```python
from build123d import *

# Parameters (mm, degrees)
RESSALTO_EXTRUS_O1_DEPTH      = 13.75
RESSALTO_EXTRUS_O1_DEPTH_BACK = 13.75
CORTE_EXTRUS_O1_DEPTH         = 13.75
CORTE_EXTRUS_O1_DEPTH_BACK    = 13.75
ESBO_O1_W                     = 2.8
ESBO_O1_H                     = 2.8
CORTE_EXTRUS_O2_DEPTH         = 13.75
CORTE_EXTRUS_O2_DEPTH_BACK    = 13.75


with BuildPart() as part:
    # Esboço2 → Ressalto-extrusão1 (new, two sides: drawn at the far end of the back side and taken through both)
    with BuildSketch(Plane(origin=(0, 0, 0), x_dir=(0, 0, -1), z_dir=(1, 0, 0)).offset(-RESSALTO_EXTRUS_O1_DEPTH_BACK)):
        with BuildLine():
            Line((2, 3.464101615), (2, -3.464101615))
            ThreePointArc((2, -3.464101615), (-4, 0), (2, 3.464101615))
        make_face()
    extrude(amount=RESSALTO_EXTRUS_O1_DEPTH + RESSALTO_EXTRUS_O1_DEPTH_BACK)

    # Esboço1 → Corte-extrusão1 (cut, two sides: drawn at the far end of the back side and taken through both)
    with BuildSketch(Plane.XY.offset(-CORTE_EXTRUS_O1_DEPTH_BACK)):
        with Locations((9.75, 0)):
            Rectangle(ESBO_O1_W, ESBO_O1_H)
        with BuildLine():
            Line((9.75, 4), (9.75, 5))
            Line((9.75, 5), (14.75, 5))
            Line((14.75, 5), (14.75, -5))
            Line((14.75, -5), (9.75, -5))
            Line((9.75, -5), (9.75, -4))
            ThreePointArc((9.75, -4), (13.75, 0), (9.75, 4))
        make_face()
        with BuildLine():
            Line((-9.75, -4), (-9.75, -5))
            Line((-9.75, -5), (-14.75, -5))
            Line((-14.75, -5), (-14.75, 5))
            Line((-14.75, 5), (-9.75, 5))
            Line((-9.75, 5), (-9.75, 4))
            ThreePointArc((-9.75, 4), (-13.75, 0), (-9.75, -4))
        make_face()
        with Locations((-9.75, 0)):
            Rectangle(ESBO_O1_W, ESBO_O1_H)
    extrude(amount=CORTE_EXTRUS_O1_DEPTH + CORTE_EXTRUS_O1_DEPTH_BACK, mode=Mode.SUBTRACT)

    # Esboço3 → Corte-extrusão2 (cut, two sides: drawn at the far end of the back side and taken through both)
    with BuildSketch(Plane(origin=(0, 0, 0), x_dir=(1, 0, 0), z_dir=(0, 1, 0)).offset(-CORTE_EXTRUS_O2_DEPTH_BACK)):
        Polygon((-7, -2.746998799), (-5.75, -4), (-5.75, -4.746998799), (-13.75, -4.746998799), (-13.75, -2.746998799), align=None)
        Polygon((13.75, -4.746998799), (13.75, -2.746998799), (7, -2.746998799), (5.75, -4), (5.75, -4.746998799), align=None)
    extrude(amount=CORTE_EXTRUS_O2_DEPTH + CORTE_EXTRUS_O2_DEPTH_BACK, mode=Mode.SUBTRACT)


solid = part.part
```
Here's how the part is built. I have some questions about the finished solid (model axes, mm). A direction names the side the tool comes from. Give positions to 0.01 mm unless a question says otherwise; leave off trailing zeros. Write each loop counter-clockwise with the first axis right and the second up, starting at its lowest first coordinate (ties: lowest second). Pieces come first, ordered by that corner, then holes.
(1) Imagine slicing it at A-A, the plane y = 0.75. Write out the boundary of the cut face in (x, z).
Output values:
outline: (-13.68, -2) - (-11.15, -2) - (-11.15, 2.75) - (-13.68, 2.75) - close; (-8.35, -2) - (8.35, -2) - (8.35, 2.75) - (7, 2.75) - (5.82, 3.93) - (-5.82, 3.93) - (-7, 2.75) - (-8.35, 2.75) - close; (11.15, -2) - (13.68, -2) - (13.68, 2.75) - (11.15, 2.75) - close
(2) Will these pins go through, and if not, where does the flat tip stop? pin 1 (0.8 mm diameter, centred on x = 9.5, z = 1.5, fed in from +Y); pin 2 (3 mm diameter, centred on x = 11, y = 1, fed in from +Z); pin 3 (1.5 mm diameter, centred on y = -2.5, z = 2, fed in from -X); pin 4 (0.8 mm diameter, centred on y = 0.5, z = 1.5, fed in from +X).
Output values:
pin 1: stops at y = 3.85
pin 2: stops at z = 2.75
pin 3: stops at x = -13.35
pin 4: stops at x = 13.75
(3) Thinking about a two-plate mould opening in X: for faces 1 (the face through (10, 1.4, 0)), 2 (the face through (0, 0, 4)), 3 (the face through (-13.75, 0.09, 0.34)), 4 (the face through (8.35, 0, 0)), which applies, pulls with the +X half, pulls with the -X half, needs draft (parallel to the pull), parting line crosses it, or undercut?
Output values:
face 1: undercut
face 2: needs draft
face 3: pulls with the -X half
face 4: undercut
(4) On a 3-axis mill with a long thin cutter (end or side, diameter ignored), from which of +Z, -Z, +X, -X, +Y, -Y can I reach the whole of each face in a straight line? I mean faces 5 (the face through (-11.15, 0, 0)), 6 (the face through (12, 0, 2.747)), 7 (the face through (-12, 0, 2.747)). Say none if no direction works.
Output values:
face 5: +Z, -Z
face 6: +Z, +X, +Y, -Y
face 7: +Z, -X, +Y, -Y
(5) Imagine slicing it at D-D, the plane z = -0.5. Write out the boundary of the cut face in (x, y), and give its area (3 significant figures).
Output values:
outline: (-10.25, -3.97) - (10.25, -3.97) arc R4 ccw to (10.25, 3.97) - (-10.25, 3.97) arc R4 ccw to start; hole (-11.15, -1.4) - (-8.35, -1.4) - (-8.35, 1.4) - (-11.15, 1.4) - close; hole (8.35, -1.4) - (11.15, -1.4) - (11.15, 1.4) - (8.35, 1.4) - close
area: 189 mm2
(6) If I drill on L1, parallel to X at y = 0, z = -0.5; L2, parallel to X at y = 1, z = 1.5; L3, parallel to Z at x = 9.75, y = 1.5, over which ranges is the centre line in solid material (lowest first)?
Output values:
L1: x = -13.75 to -11.15, -8.35 to 8.35, 11.15 to 13.75
L2: x = -13.62 to -11.15, -8.35 to 8.35, 11.15 to 13.62
L3: z = -2 to 2.75
(7) Imagine slicing it at C-C, the plane y = 2.5. Write out the boundary of the cut face in (x, z), and give its area (3 significant figures).
Output values:
outline: (-12.87, -2) - (12.87, -2) - (12.87, 2.75) - (7, 2.75) - (6.63, 3.12) - (-6.63, 3.12) - (-7, 2.75) - (-12.87, 2.75) - close
area: 127 mm2
(8) Imagine slicing it at B-B, the plane z = 1. Write out the boundary of the cut face in (x, y), and give its area (3 significant figures).
Output values:
outline: (-10.75, -3.87) - (10.75, -3.87) arc R4 ccw to (10.75, 3.87) - (-10.75, 3.87) arc R4 ccw to start; hole (-11.15, -1.4) - (-8.35, -1.4) - (-8.35, 1.4) - (-11.15, 1.4) - close; hole (8.35, -1.4) - (11.15, -1.4) - (11.15, 1.4) - (8.35, 1.4) - close
area: 185 mm2
